The drawing under review shows one solid part. Ordinate dimensions are in mm from its lowest x, y, z. A direction names the side the tool comes from. Give positions to 0.01 mm unless a question says otherwise; leave off trailing zeros. Loops run counter-clockwise (first coordinate to the right, second up) from the corner with the lowest first, then second, coordinate; pieces in that order, holes last.
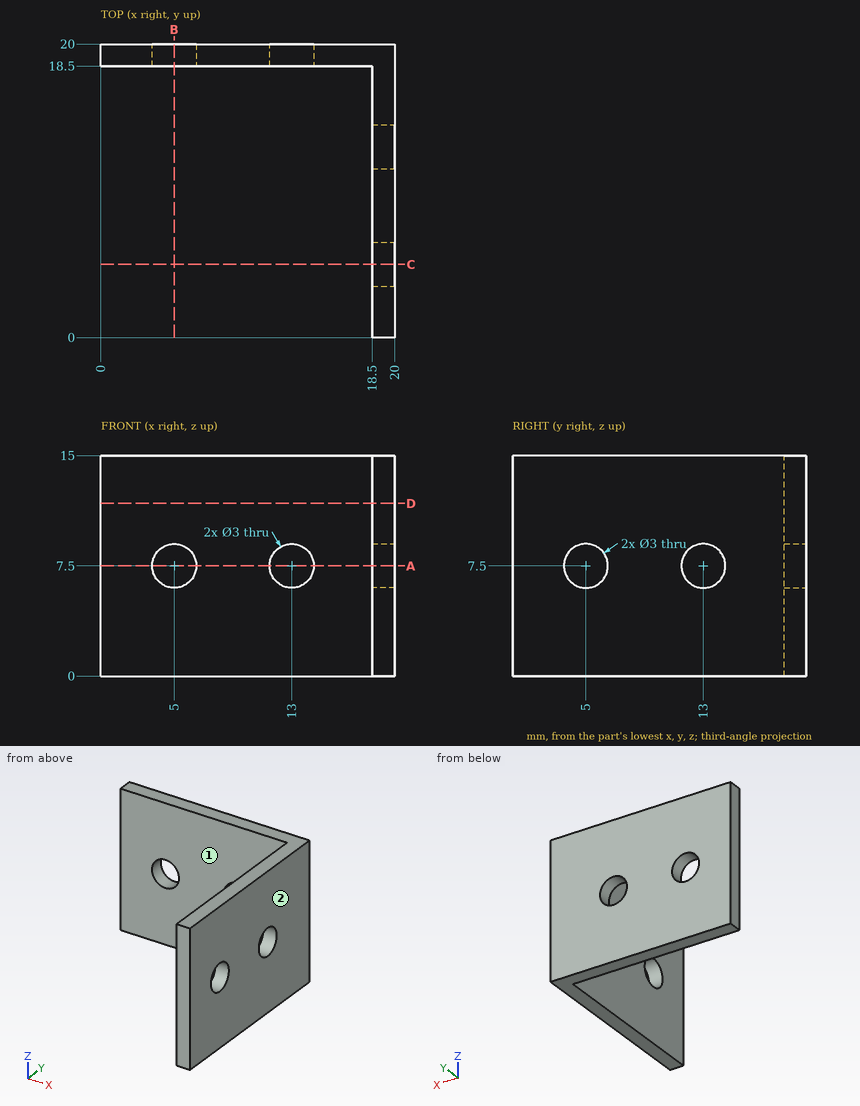
Item 1: Take a section at A-A on z = 7.5. Give the boundary of the cut face in (x, y), and give its area (4 significant figures).
Answer:
outline: (0, 18.5) - (3.5, 18.5) - (3.5, 20) - (0, 20) - close; (6.5, 18.5) - (11.5, 18.5) - (11.5, 20) - (6.5, 20) - close; (14.5, 18.5) - (18.5, 18.5) - (18.5, 14.5) - (20, 14.5) - (20, 20) - (14.5, 20) - close; (18.5, 0) - (20, 0) - (20, 3.5) - (18.5, 3.5) - close; (18.5, 6.5) - (20, 6.5) - (20, 11.5) - (18.5, 11.5) - close
area: 39.75 mm2
Item 2: Tool access review of the marked faces 1 and 2: name each direction out of +Z, -Z, +X, -X, +Y, -Y from which nothing blocks a thin tool from reaching the whole face with its end or side.
Answer:
face 1: +Z, -Z, -X, -Y
face 2: +Z, -Z, +X, +Y, -Y
Item 3: Take a section at D-D on z = 11.75. Give the boundary of the cut face in (x, y).
Answer:
outline: (0, 18.5) - (18.5, 18.5) - (18.5, 0) - (20, 0) - (20, 20) - (0, 20) - close
Item 4: For L1, parallel to Y at x = 19.25, z = 7.5; L2, parallel to Z at x = 5, y = 19.2; L3, parallel to X at y = 12.5, z = 3, list the stretches that pass through material, from the lowest coordinate up.
Answer:
L1: y = 0 to 3.5, 6.5 to 11.5, 14.5 to 20
L2: z = 0 to 6, 9 to 15
L3: x = 18.5 to 20
Item 5: Clearance check with flat-ended pins moving along their axes: pin 1 Ø4.5 at (y, z) = (8.5, 11) entering from -X; pin 2 Ø5 at (x, z) = (4, 2.5) entering from -Y; pin 3 Ø4 at (x, z) = (13, 7.5) entering from +Y. State where each tip first meets the part, or that it passes through.
Answer:
pin 1: stops at x = 18.5
pin 2: stops at y = 18.5
pin 3: stops at y = 20
Item 6: Take a section at B-B on x = 5. Give the boundary of the cut face in (y, z), and give its area (3 significant figures).
Answer:
outline: (18.5, 0) - (20, 0) - (20, 6) - (18.5, 6) - close; (18.5, 9) - (20, 9) - (20, 15) - (18.5, 15) - close
area: 18.0 mm2
